The model under review builds one solid part; all positions refer to its coordinate system, in mm. Give positions to 0.01 mm unless a question says otherwise; leave off trailing zeros. Loops run counter-clockwise (first coordinate to the right, second up) from the corner with the lowest first, then second, coordinate; pieces in that order, holes last. Notation, with made-up numbers: M 31,18.5 L 57,18.5 A14 ccw 57,42.5 Z; hole C -25,38.5 d4. An arc over 180 degrees is marked long. Return JSON: item names as keys, results as strings. Group by question number.
```python
from build123d import *

# Parameters (mm, degrees)
SKETCH1_W                      = 220
SKETCH1_H                      = 300
BOSS_EXTRUDE1_DEPTH            = 6
F_10_0_10_DIAMETER_HOLE1_D     = 10
F_10_0_10_DIAMETER_HOLE1_DEPTH = 11
F_10_0_10_DIAMETER_HOLE1_TIP   = 3.004303095


with BuildPart() as part:
    # Sketch1 → Boss-Extrude1 (new body)
    with BuildSketch(Plane(origin=(0, 0, 0), x_dir=(1, 0, 0), z_dir=(0, 1, 0))):
        Rectangle(SKETCH1_W, SKETCH1_H)
    extrude(amount=BOSS_EXTRUDE1_DEPTH)

    # Ø10.0 (10) Diameter Hole1
    with Locations(Plane.XZ):
        with Locations((-70, 117.650973616), (80, 117.650973616), (80, -22.349026384), (-70, -22.349026384)):
            Hole(F_10_0_10_DIAMETER_HOLE1_D / 2, depth=F_10_0_10_DIAMETER_HOLE1_DEPTH)
            with Locations((0, 0, -(F_10_0_10_DIAMETER_HOLE1_DEPTH + F_10_0_10_DIAMETER_HOLE1_TIP / 2))):  # 118° drill point
                Cone(0, F_10_0_10_DIAMETER_HOLE1_D / 2, F_10_0_10_DIAMETER_HOLE1_TIP, mode=Mode.SUBTRACT)


solid = part.part
```
(1) For probe 1 along Z at (x, y) = (80, 2.35), list the stretches that pass through material, from the lowest coordinate up.
(2) Add section A-A (x = -70). Write out the cut boundary in (y, z), and give its area (3 significant figures).
(3) Mouldability with a two-part tool opening along Z and no side actions: class faces 1 (the flat face through (-2, 3, 150)), 2 (the cylindrical face through (75.23, 3.04, -20.85)), 3 (the flat face through (-2, 6, -2)) as released by +Z, released by -Z, zero draft, split by the parting line, or undercut.
Verdict:
{
 "1": {"probe 1": "z = -150 to -27.35, -17.35 to 112.65, 122.65 to 150"},
 "2": {"outline": "M 0,-150 L 6,-150 L 6,-27.35 L 0,-27.35 Z; M 0,-17.35 L 6,-17.35 L 6,112.65 L 0,112.65 Z; M 0,122.65 L 6,122.65 L 6,150 L 0,150 Z", "area": "1,680 mm²"},
 "3": {"face 1": "released by +Z", "face 2": "undercut", "face 3": "zero draft"}
}
